Check sheet for the modelled part. Datum: model origin and axes. Units: mm. Face numbers are marked on the shaded views. A direction names the side the tool comes from. Round coordinates to 2 decimals unless told otherwise and drop trailing zeros. Order: outer loops, then holes, each group sorted by start corner. A loop starts at its lowest first (then second) coordinate and runs counter-clockwise, first axis right, second up.
```python
from build123d import *

# Parameters (mm, degrees)
BOSS_EXTRUDE1_DEPTH    = 2
BOSS_EXTRUDE2_DEPTH    = 10
M3_CLEARANCE_HOLE1_D   = 3.6
M2_5_CLEARANCE_HOLE1_D = 2.9


with BuildPart() as part:
    # Sketch1 → Boss-Extrude1 (new body)
    with BuildSketch(Plane(origin=(0, 0, 0), x_dir=(0, 0, -1), z_dir=(1, 0, 0))):
        Polygon((0, 0), (10, 0), (31, 21), (31, 25), (21, 25), (0, 4), align=None)
    extrude(amount=BOSS_EXTRUDE1_DEPTH)

    # Sketch2 → Boss-Extrude2 (add)
    with BuildSketch(Plane(origin=(2, 0, 0), x_dir=(0, 0, -1), z_dir=(1, 0, 0))):
        Polygon((10, 0), (0, 0), (0, 2), (8.797060967, 2), (21, 25), (31, 25), (31, 23), (22.202939033, 23), align=None)
    extrude(amount=BOSS_EXTRUDE2_DEPTH)

    # M3 Clearance Hole1 (through all)
    with Locations(Plane(origin=(0, 2, 0), x_dir=(1, 0, 0), z_dir=(0, 1, 0))):
        with Locations((6, 5)):
            Hole(M3_CLEARANCE_HOLE1_D / 2)

    # M2.5 Clearance Hole1 (through all)
    with Locations(Plane(origin=(0, 25, 0), x_dir=(1, 0, 0), z_dir=(0, 1, 0))):
        with Locations((6.5, 27)):
            Hole(M2_5_CLEARANCE_HOLE1_D / 2)

    # Mirror1: part across plane


with BuildPart() as part_1:
    add(part.part)
    add(part.part.mirror(Plane.ZY.offset(-12)))


solid = part_1.part
```
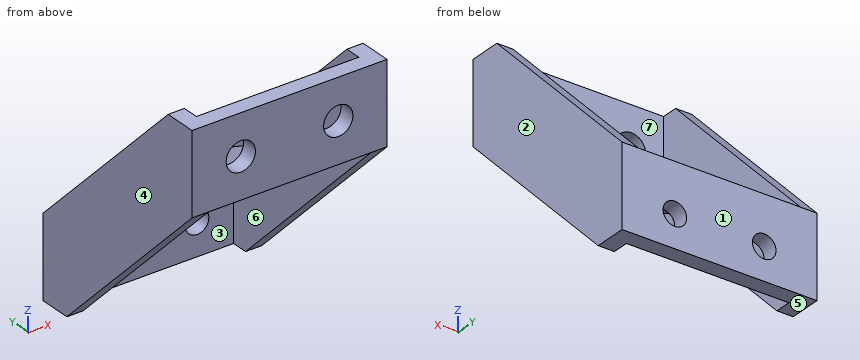
Item 1: Sectioned sample at D-D (y = 16.25). Record the cut outline in (x, z), and give its area (3 significant figures).
Answer:
outline: (0, -26.25) - (2, -26.25) - (2, -18.62) - (22, -18.62) - (22, -26.25) - (24, -26.25) - (24, -12.25) - (22, -12.25) - (22, -16.36) - (2, -16.36) - (2, -12.25) - (0, -12.25) - close
area: 101 mm2
Item 2: Sectioned sample at C-C (z = -2.5). Record the cut outline in (x, y), and give its area (3 significant figures).
Answer:
outline: (0, 0) - (24, 0) - (24, 6.5) - (22, 6.5) - (22, 2) - (2, 2) - (2, 6.5) - (0, 6.5) - close
area: 66.0 mm2
Item 3: Go/stop test with flat-tipped pins: P1, Ø8, axis at x = 21, y = 8, coming from the -Z side; P2, Ø3, axis at x = 6, z = -5, coming from the +Y side; P3, Ø4, axis at x = 16, y = 14.5, coming from the +Z side; P4, Ø4, axis at x = 14, z = -7, coming from the +Y side. Record where each tip stops, or that it passes through.
Answer:
P1: stops at z = -21.87
P2: passes through
P3: stops at z = -14.37
P4: stops at y = 2.38
Item 4: Release check for a two-part mould opening along X. For the marked faces 1, 2, 3 and 4 record: released by +X, released by -X, zero draft, split by the parting line, or undercut.
Answer:
face 1: zero draft
face 2: released by +X
face 3: undercut
face 4: released by -X
Item 5: Sectioned sample at A-A (z = -27). Record the cut outline in (x, y), and give its area (3 significant figures).
Answer:
outline: (0, 17) - (2, 17) - (2, 23) - (5.05, 23) - (5.05, 25) - (0, 25) - close; (7.95, 23) - (16.05, 23) - (16.05, 25) - (7.95, 25) - close; (18.95, 23) - (22, 23) - (22, 17) - (24, 17) - (24, 25) - (18.95, 25) - close
area: 60.4 mm2
Item 6: Scan lines: line 1 along X through (y, z) = (1.2, -5); line 2 along X through (y, z) = (23.9, -27); line 3 along X through (y, z) = (22.25, -22). Record each from-to range of solid material in increasing order.
Answer:
line 1: x = 0 to 4.2, 7.8 to 16.2, 19.8 to 24
line 2: x = 0 to 5.05, 7.95 to 16.05, 18.95 to 24
line 3: x = 0 to 2, 22 to 24
Item 7: Sectioned sample at B-B (x = 5.5). Record the cut outline in (y, z), and give its area (3 significant figures).
Answer:
outline: (0, -10) - (23, -22.2) - (23, -25.95) - (25, -25.95) - (25, -21) - (2, -8.8) - (2, -6.73) - (0, -6.73) - close; (0, -3.27) - (2, -3.27) - (2, 0) - (0, 0) - close; (23, -31) - (25, -31) - (25, -28.05) - (23, -28.05) - close
area: 78.6 mm2
Item 8: Access from +Z, -Z, +X, -X, +Y, -Y to the whole of each face (thin tool, end or side, straight path). Record for the marked faces 5, 6 and 7.
Answer:
face 5: -Z, +X, -X, +Y, -Y
face 6: -Z, -Y
face 7: +Z, +Y
